```python
from build123d import *

# Parameters (mm, degrees)
ESQUISSE1_W                                       = 25
ESQUISSE1_H                                       = 26
BOSS_EXTRU_1_DEPTH                                = 4
BOSS_EXTRU_2_DEPTH                                = 25
ESQUISSE3_R                                       = 1.5
ENL_V_MAT_EXTRU_1_DEPTH                           = 25
ESQUISSE4_W                                       = 7.6
ESQUISSE4_H                                       = 3
ESQUISSE4_H_2                                     = 6
ENL_V_MAT_EXTRU_2_DEPTH                           = 25
ENL_V_MAT_EXTRU_2_DEPTH_BACK                      = 25
CHAMBRAGE_POUR_VIS_SIX_PANS_CREUX_M41_D           = 4.2
CHAMBRAGE_POUR_VIS_SIX_PANS_CREUX_M41_CBORE_D     = 8
CHAMBRAGE_POUR_VIS_SIX_PANS_CREUX_M41_CBORE_DEPTH = 2
CONG_1_R                                          = 1


with BuildPart() as part:
    # Esquisse1 → Boss.-Extru.1 (new body)
    with BuildSketch(Plane.XY):
        with Locations((12.5, 13)):
            Rectangle(ESQUISSE1_W, ESQUISSE1_H)
    extrude(amount=BOSS_EXTRU_1_DEPTH)

    # Esquisse2 → Boss.-Extru.2 (add)
    with BuildSketch(Plane(origin=(25, 0, 0), x_dir=(0, 0, -1), z_dir=(1, 0, 0))):
        with BuildLine():
            ThreePointArc((-1, 23), (-1.878679656, 25.121320344), (-4, 26))
            Line((-4, 26), (-4, 20))
            ThreePointArc((-4, 20), (-1.878679656, 20.878679656), (-1, 23))
        make_face()
        with BuildLine():
            Line((-4, 20), (-4, 26))
            ThreePointArc((-4, 26), (-7, 23), (-4, 20))
        make_face()
    extrude(amount=-BOSS_EXTRU_2_DEPTH)

    # Esquisse3 → Enl_v. mat.-Extru.1 (cut)
    with BuildSketch(Plane(origin=(25, 0, 0), x_dir=(0, 0, -1), z_dir=(1, 0, 0))):
        with Locations((-4, 23)):
            Circle(ESQUISSE3_R)
        with BuildLine():
            ThreePointArc((-3, 26), (-0.878679656, 25.121320344), (0, 23))
            Line((0, 23), (0, 26))
            Line((0, 26), (-3, 26))
        make_face()
    extrude(amount=-ENL_V_MAT_EXTRU_1_DEPTH, mode=Mode.SUBTRACT)

    # Esquisse4 → Enl_v. mat.-Extru.2 (cut, two sides)
    with BuildSketch(Plane.XY.offset(4)) as enl_v_mat_extru_2_sk:
        with Locations((3.8, 18.5)):
            Rectangle(ESQUISSE4_W, ESQUISSE4_H)
        with Locations((3.8, 23)):
            Rectangle(ESQUISSE4_W, ESQUISSE4_H_2)
        with Locations((21.2, 23)):
            Rectangle(ESQUISSE4_W, ESQUISSE4_H_2)
        with Locations((21.2, 18.5)):
            Rectangle(ESQUISSE4_W, ESQUISSE4_H)
    extrude(amount=ENL_V_MAT_EXTRU_2_DEPTH, mode=Mode.SUBTRACT)
    extrude(enl_v_mat_extru_2_sk.sketch, amount=-ENL_V_MAT_EXTRU_2_DEPTH_BACK, mode=Mode.SUBTRACT)

    # Chambrage pour vis _ six pans creux M41 (through all)
    with Locations(Plane(origin=(5.5, 8.51504076, 4), x_dir=(1, 0, 0), z_dir=(0, 0, 1))):
        with Locations((0, 0), (14, 0)):
            CounterBoreHole(CHAMBRAGE_POUR_VIS_SIX_PANS_CREUX_M41_D / 2, CHAMBRAGE_POUR_VIS_SIX_PANS_CREUX_M41_CBORE_D / 2, CHAMBRAGE_POUR_VIS_SIX_PANS_CREUX_M41_CBORE_DEPTH)

    # Cong_1
    cong_1_edges = [part.edges().sort_by_distance(p)[0] for p in [
        (25, 8.5, 4),
        (0, 8.5, 4),
        (21.2, 17, 4),
        (3.8, 17, 4),
        (0, 8.5, 0),
        (25, 8.5, 0),
        (0, 17, 2),
        (3.8, 17, 0),
        (7.6, 26, 3.5),
        (7.6, 18.5, 4),
        (7.6, 17, 2),
        (7.6, 25.121320344, 0.878679656),
        (7.6, 20, 0),
        (7.6, 23, 7),
        (12.5, 0, 0),
        (21.2, 17, 0),
        (17.4, 17, 2),
        (17.4, 23, 7),
        (17.4, 26, 3.5),
        (17.4, 25.121320344, 0.878679656),
        (17.4, 20, 0),
        (17.4, 18.5, 4),
        (25, 17, 2),
        (25, 0, 2),
        (0, 0, 2),
        (12.5, 0, 4),
    ]]
    fillet(cong_1_edges, radius=CONG_1_R)


solid = part.part
```
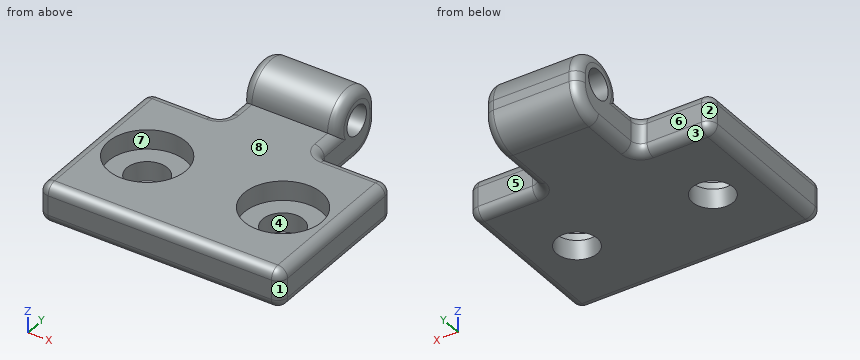
Geometry check sheet. Reference: the model listing, model coordinates, mm. Face numbers are marked on the shaded views. A direction names the side the tool comes from. Coordinates: 2 decimals unless noted, no trailing zeros. Write each loop counter-clockwise with the first axis right and the second up, starting at its lowest first coordinate (ties: lowest second). Pieces come first, ordered by that corner, then holes. Notation, with made-up numbers: M -9.75,54 L 24.25,54 A36 ccw 24.25,91 Z; hole C 89,75 d9. An arc over 180 degrees is marked long. Answer as a JSON object with one key per item and string values.
1. Draft check along X on the marked faces 1, 2, 3 and 4. Enter one of: released by +X, released by -X, zero draft, split by the parting line, or undercut.
Answers below:
{"face 1": "released by +X", "face 2": "released by -X", "face 3": "zero draft", "face 4": "undercut"}
2. Section check A-A, the plane x = 5.5. Enter the section's corners in (y, z), plus the area to 3 significant figures.
Answers below:
{"outline": "M 0,1 A1 ccw 1,0 L 6.42,0 L 6.42,2 L 4.52,2 L 4.52,4 L 1,4 A1 ccw 0,3 Z; M 10.62,0 L 16,0 A1 ccw 17,1 L 17,3 A1 ccw 16,4 L 12.52,4 L 12.52,2 L 10.62,2 Z", "area": "42.7 mm²"}
3. Go/stop test with flat-tipped pins: pin 1 Ø10 at (x, y) = (18, 9.5) entering from +Z; pin 2 Ø3 at (x, z) = (14, 2.5) entering from +Y; pin 3 Ø1.5 at (x, z) = (11.5, 6) entering from -Y; pin 4 Ø2 at (x, z) = (2.5, 2) entering from +Y. Record where each tip stops, or that it passes through.
Answers below:
{"pin 1": "stops at z = 4", "pin 2": "stops at y = 26", "pin 3": "stops at y = 20.27", "pin 4": "stops at y = 17"}
4. Section check C-C, the plane x = 3. Enter the section's corners in (y, z), plus the area to 3 significant figures.
Answers below:
{"outline": "M 0,1 A1 ccw 1,0 L 16,0 A1 ccw 17,1 L 17,3 A1 ccw 16,4 L 11.64,4 L 11.64,2 L 5.39,2 L 5.39,4 L 1,4 A1 ccw 0,3 Z", "area": "54.7 mm²"}
5. Scan lines: L1, parallel to Y at x = 19.5, z = 1.1; L2, parallel to Z at x = 12.5, y = 23; L3, parallel to Y at x = 19.5, z = 2.5. Record each from-to range of solid material in increasing order.
Answers below:
{"L1": "y = 0 to 6.42, 10.62 to 17", "L2": "z = 0 to 2.5, 5.5 to 7", "L3": "y = 0 to 4.52, 12.52 to 17"}
6. Tool access check on the marked faces 5, 6, 7 and 8. Record the directions out of +Z, -Z, +X, -X, +Y, -Y that give a thin tool (end or side, any length) a straight path to the whole face; none if there is none.
Answers below:
{"face 5": "+Z, -Z, +X, +Y", "face 6": "+Z, -Z, -X, +Y", "face 7": "+Z", "face 8": "+Z, +X, -X, -Y"}
7. Section check B-B, the plane x = 13. Enter the section's corners in (y, z).
Answers below:
{"outline": "M 0,1 A1 ccw 1,0 L 23,0 A3 ccw 26,3 L 26,4 A3 ccw 20,4 L 1,4 A1 ccw 0,3 Z; hole C 23,4 d3"}
